Read the model definition and answer for the solid it produces. Units are mm, in the model's axes. Face numbers are marked on the shaded views. Coordinates: 2 decimals unless noted, no trailing zeros. Write each loop counter-clockwise with the first axis right and the second up, starting at its lowest first coordinate (ties: lowest second). Pieces come first, ordered by that corner, then holes. Notation, with made-up numbers: (-10.5, 58) -> (34.5, 58) arc R18 ccw to (34.5, 72) -> close; hole circle Ø1 at (88.25, 19.25). An arc over 180 degrees is marked (long way). One line per item, written item: value. Start each with the question number.
1. For a pull along Y with two mould halves and no side action, classify the marked faces 1 and 2 as pulls with the +Y half, pulls with the -Y half, needs draft (parallel to the pull), parting line crosses it, or undercut.
2. Find section A-A, the plane y = 0. Write down the section's boundary in (x, z).
3. Find section D-D, the plane x = -10.5. Write down the section's boundary in (y, z).
4. Find section C-C, the plane x = 1.25. Write down the section's boundary in (y, z).
5. Consider line 1 along Y through (x, z) = (-1.75, 6); line 2 along X through (y, z) = (7.5, 6.2); line 3 along Y through (x, z) = (5.5, 6.9). Determine where each line is inside the solid, lowest interval first.
6. Given P1, Ø1.5, axis at y = 8, z = 7.5, coming from the +X side, flat-ended and moving along its own axis, determine where the tip first touches the part or whether it passes through.
7. Find section B-B, the plane z = 6.2. Write down the section's boundary in (x, y).
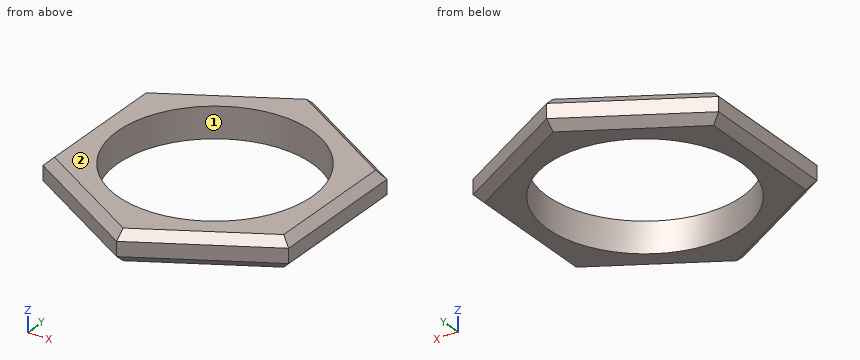
```python
from build123d import *

# Parameters (mm, degrees)
SKETCH019_R     = 9.5
PAD009_DEPTH    = 3
CHAMFER005_SIZE = 0.8
CHAMFER004_SIZE = 0.8


with BuildPart() as part:
    # Sketch019 → Pad009 (new body)
    with BuildSketch(Plane.XY):
        Polygon((12, -6.928203), (12, 6.928203), (0, 13.856406), (-12, 6.928203), (-12, -6.928203), (0, -13.856406), align=None)
        Circle(SKETCH019_R, mode=Mode.SUBTRACT)
    extrude(amount=PAD009_DEPTH)

    # Chamfer005
    chamfer005_edges = [part.edges().sort_by_distance(p)[0] for p in [
        (12, 0, 3),
        (6, -10.392305, 3),
        (-6, -10.392305, 3),
        (-12, 0, 3),
        (-6, 10.392305, 3),
        (6, 10.392305, 3),
    ]]
    chamfer(chamfer005_edges, length=CHAMFER005_SIZE)

    # Chamfer004
    chamfer004_edges = [part.edges().sort_by_distance(p)[0] for p in [
        (-6, 10.392305, 0),
        (-12, 0, 0),
        (-6, -10.392305, 0),
        (6, -10.392305, 0),
        (12, 0, 0),
        (6, 10.392305, 0),
    ]]
    chamfer(chamfer004_edges, length=CHAMFER004_SIZE)


with BuildPart() as part_1:
    # Body006 placement: moved
    add(part.part.moved(Location((0, 0, 5))))


solid = part_1.part
```
Answer block:
1. face 1: undercut
1. face 2: needs draft
2. outline: (-12, 5.8) -> (-11.2, 5) -> (-9.5, 5) -> (-9.5, 8) -> (-11.2, 8) -> (-12, 7.2) -> close; (9.5, 5) -> (11.2, 5) -> (12, 5.8) -> (12, 7.2) -> (11.2, 8) -> (9.5, 8) -> close
3. outline: (-7.79, 5.8) -> (-6.87, 5) -> (6.87, 5) -> (7.79, 5.8) -> (7.79, 7.2) -> (6.87, 8) -> (-6.87, 8) -> (-7.79, 7.2) -> close
4. outline: (-13.13, 5.8) -> (-12.21, 5) -> (-9.42, 5) -> (-9.42, 8) -> (-12.21, 8) -> (-13.13, 7.2) -> close; (9.42, 5) -> (12.21, 5) -> (13.13, 5.8) -> (13.13, 7.2) -> (12.21, 8) -> (9.42, 8) -> close
5. line 1: y = -12.85 to -9.34, 9.34 to 12.85
5. line 2: x = -11.01 to -5.83, 5.83 to 11.01
5. line 3: y = -10.68 to -7.75, 7.75 to 10.68
6. P1: stops at x = 11.33
7. outline: (-12, -6.93) -> (0, -13.86) -> (12, -6.93) -> (12, 6.93) -> (0, 13.86) -> (-12, 6.93) -> close; hole circle Ø19 at (0, 0)
